```python
from build123d import *

# Parameters (mm, degrees)
BOSS_EXTRUDE2_START = 3
SKETCH3_R           = 18.5
SKETCH3_R_2         = 2
SKETCH3_R_3         = 11.496935192
BOSS_EXTRUDE2_DEPTH = 3


# Read off the part's stored shape, not the designer's step: Revolve1
with BuildPart() as part:
    # Revolve1 outline → Revolve1 (revolve)
    with BuildSketch(Plane.XY):
        Polygon((26.378679656, 0), (22, 4.378679656), (22, 16), (18.5, 16), (18.5, -16), (22, -16), (22, -4.378679656), align=None)
    revolve(axis=Axis((0, 0, 0), (0, 1, 0)))

    # Sketch3 → Boss-Extrude2 (add)
    with BuildSketch(Plane.XZ.offset(-16).offset(BOSS_EXTRUDE2_START)):
        with Locations(Location((0, 0, 0), (0, 0, 270))):
            Circle(SKETCH3_R)
        with Locations(Location((15, 0, 0), (0, 0, 270))):
            Circle(SKETCH3_R_2, mode=Mode.SUBTRACT)
        with Locations(Location((0, 0, 0), (0, 0, 270))):
            Circle(SKETCH3_R_3, mode=Mode.SUBTRACT)
        with Locations(Location((0, -15, 0), (0, 0, 270))):
            Circle(SKETCH3_R_2, mode=Mode.SUBTRACT)
        with Locations(Location((-15, 0, 0), (0, 0, 270))):
            Circle(SKETCH3_R_2, mode=Mode.SUBTRACT)
        with Locations(Location((0, 15, 0), (0, 0, 270))):
            Circle(SKETCH3_R_2, mode=Mode.SUBTRACT)
    extrude(amount=-BOSS_EXTRUDE2_DEPTH)


solid = part.part
```
Source: CAD feature listing. Evaluate the final solid. Frame: model axes, mm. A direction names the side the tool comes from. Round coordinates to 2 decimals unless told otherwise and drop trailing zeros. Loops run counter-clockwise (first coordinate to the right, second up) from the corner with the lowest first, then second, coordinate; pieces in that order, holes last. Notation, with made-up numbers: M 37.25,76.25 L 54.25,76.25 A37 cw 54.25,114.25 Z; hole C -38.5,-2.75 d8. An arc over 180 degrees is marked long. Use a Markdown table: item, result. Add a question column.
1. Reachability of faces 1 (the cylindrical face through (-4.769, 10.271, 21.477)), 2 (the flat face through (8.5, 13, -8)), 3 (the cylindrical face through (-13, 14, 0)) from +Z, -Z, +X, -X, +Y, -Y: full face, straight path, thin tool, end or side. Return the list, or none.
2. Line query: line 1 (X direction, y = 15, z = 0); line 2 (X direction, y = 12, z = 0); line 3 (X direction, y = 8.5, z = -2). Output: solid intervals per line, ascending.
3. Section query C-C on y = -3.5. Return the cut outline in (x, z), then the cut area to 3 significant figures.
4. Section query A-A on y = -14. Return the cut outline in (x, z).
5. Mould query, pull axis Z, two halves, no side actions, for faces 4 (the cylindrical face through (-4.01, -1.7, 18.06)), 5 (the conical face through (-4.829, -4.105, 21.744)), 6 (the flat face through (-9, 16, -9)), 7 (the cylindrical face through (-1.2, 14.5, 16.6)). Classes: pulls with the +Z half, pulls with the -Z half, needs draft (parallel to the pull), parting line crosses it, or undercut.
6. Contact query for flat-ended pins moving along their axis: P1, Ø6, axis at y = 0, z = 11.5, coming from the -X side; P2, Ø8, axis at y = -10, z = 5.5, coming from the +X side; P3, Ø5, axis at x = 15, z = 0, coming from the -Y side; P4, Ø5, axis at x = -15, z = 0, coming from the +Y side. Output: stop coordinate, or through.
7. Section query B-B on z = -1. Give the number of separate pieces and of enclosed holes in the cut face, then the cut area to 3 significant figures.
Reported:
| question | item | result |
|---|---|---|
| 1 | face 1 | +Y |
| 1 | face 2 | -Y |
| 1 | face 3 | +Y, -Y |
| 2 | line 1 | x = -22 to -17, -13 to -11.5, 11.5 to 13, 17 to 22 |
| 2 | line 2 | x = -22 to -18.5, 18.5 to 22 |
| 2 | line 3 | x = -21.91 to -18.39, 18.39 to 21.91 |
| 3 | outline | C 0,0 d45.76; hole C 0,0 d37 |
| 3 | area | 569 mm² |
| 4 | outline | C 0,0 d44; hole C 0,0 d37 |
| 5 | face 4 | undercut |
| 5 | face 5 | parting line crosses it |
| 5 | face 6 | needs draft |
| 5 | face 7 | undercut |
| 6 | P1 | stops at x = -24.97 |
| 6 | P2 | stops at x = 21.95 |
| 6 | P3 | stops at y = 13 |
| 6 | P4 | stops at y = 16 |
| 7 | separate pieces | 4 |
| 7 | enclosed holes | 0 |
| 7 | area | 284 mm² |
